Input: part model. Units: mm. Frame: model coordinates. Coordinates: 2 decimals unless noted, no trailing zeros. Loops run counter-clockwise (first coordinate to the right, second up) from the corner with the lowest first, then second, coordinate; pieces in that order, holes last.
(1) Mould query, pull axis Y, two halves, no side actions, for faces 1 (the face through (4, -1, -35)), 2 (the face through (4.06, 44.49, 32.15)), 3 (the face through (3.9, 35.6, 15)). Classes: released by +Y, released by -Y, zero draft, split by the parting line, or undercut.
(2) Section B-B, the plane y = 35.5. Return loops of the section in (x, z).
(3) Section C-C, the plane z = -17.5. Return loops of the section in (x, y).
(4) Line query: L1, parallel to Y at x = 6.75, z = -17.5; L2, parallel to Y at x = 5, z = -19.5; L3, parallel to Z at x = 5.75, y = 36. Output: solid intervals per line, ascending.
(5) Section A-A, the plane x = 5. Return loops of the section in (y, z), then the cut area to 3 significant figures.
(6) Contact query for a flat-ended pin moving along its axis: P1, Ø8, axis at y = 35.5, z = -17.5, coming from the +X side. Output: stop coordinate, or through.
```python
from build123d import *

# Parameters (mm, degrees)
SKETCH_1_W             = 70
SKETCH_1_H             = 95
EXTRUDE_1_DEPTH        = 8
HOLE_WIZARD_M6_1_D     = 5
HOLE_WIZARD_M6_1_DEPTH = 17
HOLE_WIZARD_M6_1_TIP   = 1.502151548
FILLET_1_R             = 10


with BuildPart() as part:
    # 草图1 → 凸台-拉伸1 (new body)
    with BuildSketch(Plane(origin=(0, 0, 0), x_dir=(0, 0, -1), z_dir=(1, 0, 0))):
        Rectangle(SKETCH_1_W, SKETCH_1_H)
    extrude(amount=EXTRUDE_1_DEPTH)

    # M6 螺纹孔1
    with Locations(Plane(origin=(8, 0, 0), x_dir=(0, 0, -1), z_dir=(1, 0, 0))):
        with Locations((-17.5, 35.5), (17.5, 35.5), (-17.5, -19.5), (17.5, -19.5)):
            Hole(HOLE_WIZARD_M6_1_D / 2, depth=HOLE_WIZARD_M6_1_DEPTH)
            with Locations((0, 0, -(HOLE_WIZARD_M6_1_DEPTH + HOLE_WIZARD_M6_1_TIP / 2))):  # 118° drill point
                Cone(0, HOLE_WIZARD_M6_1_D / 2, HOLE_WIZARD_M6_1_TIP, mode=Mode.SUBTRACT)

    # 圆角1
    fillet_1_edges = [part.edges().sort_by_distance(p)[0] for p in [
        (4, 47.5, 35),
        (4, 47.5, -35),
        (4, -47.5, -35),
        (4, -47.5, 35),
    ]]
    fillet(fillet_1_edges, radius=FILLET_1_R)


solid = part.part
```
Report:
1. face 1: zero draft
1. face 2: released by +Y
1. face 3: undercut
2. outline: (0, -35) - (8, -35) - (8, -20) - (0, -20) - close; (0, -15) - (8, -15) - (8, 15) - (0, 15) - close; (0, 20) - (8, 20) - (8, 35) - (0, 35) - close
3. outline: (0, -47.5) - (8, -47.5) - (8, -22) - (0, -22) - close; (0, -17) - (8, -17) - (8, 33) - (0, 33) - close; (0, 38) - (8, 38) - (8, 47.5) - (0, 47.5) - close
4. L1: y = -47.5 to -22, -17 to 33, 38 to 47.5
4. L2: y = -47.5 to -21, -18 to 34, 37 to 47.5
4. L3: z = -35 to -19.95, -15.05 to 15.05, 19.95 to 35
5. outline: (-47.5, -25) arc R10 ccw to (-37.5, -35) - (37.5, -35) arc R10 ccw to (47.5, -25) - (47.5, 25) arc R10 ccw to (37.5, 35) - (-37.5, 35) arc R10 ccw to (-47.5, 25) - close; hole circle Ø5 at (-19.5, -17.5); hole circle Ø5 at (-19.5, 17.5); hole circle Ø5 at (35.5, -17.5); hole circle Ø5 at (35.5, 17.5)
5. area: 6,490 mm2
6. P1: stops at x = 8
